Read the model definition and answer for the solid it produces. Units are mm, in the model's axes. A direction names the side the tool comes from. Coordinates: 2 decimals unless noted, no trailing zeros. Loops run counter-clockwise (first coordinate to the right, second up) from the corner with the lowest first, then second, coordinate; pieces in that order, holes last. Notation, with made-up numbers: (30, -39.75) - (88, -39.75) arc R33 cw to (88, -4.75) - close; hole circle Ø11 at (43, 10). An arc over 180 degrees is marked (long way). Use one line per item in the form item = value.
Autodesk Inventor part; units mm, degrees
ref_plane "Work Plane1" through (0, 0, 4.4125) normal (0, 0, 1) x (1, 0, 0)
ref_plane "YZ Plane" through (0, 0, 0) normal (1, 0, 0) x (0, 1, 0)
ref_plane "XZ Plane" through (0, 0, 0) normal (0, 1, 0) x (-1, 0, 0)
sketch "Sketch4" plane through (0, 0, 0) normal (0, 1, 0) x (-1, 0, 0)
  line L0 (0, 0) -> (6.5, 0) construction
  line L1 (6.5, 0) -> (6.5, -9.525)
  line L2 (6.5, -9.525) -> (0, -9.525)
  line L3 (0, -9.525) -> (0, 0)
  line L4 (0, -9.525) -> (19.05, -9.525)
  line L5 (19.05, -9.525) -> (19.05, 0) construction
  line L6 (19.05, 0) -> (0, 0)
  line L7 (0, 0) -> (0, -9.525) construction
  line L8 (19.05, 0) -> (16.9384, -9.525)
  line L9 (17.424, 0) -> (15.3123, -9.525)
  line L10 (15.6643, -7.9375) -> (6.5, -7.9375)
  line L11 (6.5, -7.9375) -> (7.5, -7.9375)
  line L12 (7.5, -7.9375) -> (7.5, -5.9375)
  line L13 (7.5, -5.9375) -> (6.5, -5.9375)
  line L14 (6.5, -5.9375) -> (6.5, -7.9375)
  line L15 (6.5, 0) -> (0, 0)
  line L16 (0, 0) -> (0, 6.35)
  line L17 (0, 6.35) -> (6.5, 6.35)
  line L18 (6.5, 6.35) -> (6.5, 0)
  line L19 (6.5, -3.175) -> (17.072, -3.175)
  line L20 (17.072, -3.175) -> (17.072, -1.5875) construction
  line L21 (17.072, -1.5875) -> (6.5, -1.5875)
  line L22 (6.5, -1.5875) -> (6.5, -3.175)
  line L23 (6.5, -3.175) -> (0, -3.175)
  line L24 (6.5, -1.5875) -> (7.5, -1.5875)
  line L25 (7.5, -1.5875) -> (7.5, 0.4125)
  line L26 (7.5, 0.4125) -> (6.5, 0.4125)
  line L27 (6.5, 0.4125) -> (6.5, -1.5875)
  line L28 (15.3123, -9.525) -> (15.3123, -3.175)
  point P0 (0, -3.175)
  point P1 (16.7201, -3.175)
  dimension "d28" = 6.5
  dimension "d30" = 19.05
  dimension "d31" = 9.525
  dimension "d32" = 12.5
  dimension "d33" = 1.5875
  dimension "d34" = 1.5875
  dimension "d36" = 1
  dimension "d37" = 2
  dimension "d53" = 6.35
  dimension "d54" = 1.5875
  dimension "d55" = 9.525
  dimension "d56" = 1
  dimension "d57" = 2
revolve "Revolution1" add sketch "Sketch4" angle 360 about axis through (0, 0, -9.525) along (0, 0, 1) contours L6 L25 L21 L1 | L1 L23 L3 L6 | L18 L26 L25 L6 | L6 L16 L17 L18 | L21 L9 L19 L1 | L6 L8 L4 L9 | L19 L9 L10 L28 | L10 L9 L28
sketch "Sketch5" plane through (0, 0, 0) normal (0, 0, 1) x (1, 0, 0)
  circle A0 centre (0, 0) radius 4.7625 construction
  line L0 (0, 0) -> (0, 4.7625) construction
  line L1 (2.7496, 4.7625) -> (5.4993, 0)
  line L2 (5.4993, 0) -> (2.7496, -4.7625)
  line L3 (2.7496, -4.7625) -> (-2.7496, -4.7625)
  line L4 (-2.7496, -4.7625) -> (-5.4993, 0)
  line L5 (-5.4993, 0) -> (-2.7496, 4.7625)
  line L6 (-2.7496, 4.7625) -> (2.7496, 4.7625)
  line L7 (-2.7496, 4.7625) -> (0, 0) construction
  arc A1 (-0.9165, 4.4712) -> (-2.6268, 4.5498) centre (-1.8331, 3.175) ccw
  arc A2 (-0.9165, 4.4712) -> (0, 4.1799) centre (0, 5.7674) ccw
  arc A3 (2.6268, 4.5498) -> (0.9165, 4.4712) centre (1.8331, 3.175) ccw
  arc A4 (0, 4.1799) -> (0.9165, 4.4712) centre (0, 5.7674) ccw
  arc A5 (-4.3304, 1.4418) -> (-5.2537, 0) centre (-3.6662, 0) ccw
  arc A6 (-4.3304, 1.4418) -> (-3.6199, 2.0899) centre (-4.9947, 2.8837) ccw
  arc A7 (-3.6199, 2.0899) -> (-3.4139, 3.0293) centre (-4.9947, 2.8837) ccw
  arc A8 (-2.6268, 4.5498) -> (-3.4139, 3.0293) centre (-1.8331, 3.175) ccw
  arc A9 (-3.4139, -3.0293) -> (-2.6268, -4.5498) centre (-1.8331, -3.175) ccw
  arc A10 (-3.4139, -3.0293) -> (-3.6199, -2.0899) centre (-4.9947, -2.8837) ccw
  arc A11 (-3.6199, -2.0899) -> (-4.3304, -1.4418) centre (-4.9947, -2.8837) ccw
  arc A12 (-5.2537, 0) -> (-4.3304, -1.4418) centre (-3.6662, 0) ccw
  arc A13 (0.9165, -4.4712) -> (2.6268, -4.5498) centre (1.8331, -3.175) ccw
  arc A14 (0.9165, -4.4712) -> (0, -4.1799) centre (0, -5.7674) ccw
  arc A15 (0, -4.1799) -> (-0.9165, -4.4712) centre (0, -5.7674) ccw
  arc A16 (-2.6268, -4.5498) -> (-0.9165, -4.4712) centre (-1.8331, -3.175) ccw
  arc A17 (4.3304, -1.4418) -> (5.2537, 0) centre (3.6662, 0) ccw
  arc A18 (4.3304, -1.4418) -> (3.6199, -2.0899) centre (4.9947, -2.8837) ccw
  arc A19 (3.6199, -2.0899) -> (3.4139, -3.0293) centre (4.9947, -2.8837) ccw
  arc A20 (2.6268, -4.5498) -> (3.4139, -3.0293) centre (1.8331, -3.175) ccw
  arc A21 (3.4139, 3.0293) -> (2.6268, 4.5498) centre (1.8331, 3.175) ccw
  arc A22 (3.4139, 3.0293) -> (3.6199, 2.0899) centre (4.9947, 2.8837) ccw
  arc A23 (3.6199, 2.0899) -> (4.3304, 1.4418) centre (4.9947, 2.8837) ccw
  arc A24 (5.2537, 0) -> (4.3304, 1.4418) centre (3.6662, 0) ccw
  point P0 (-1.8331, 4.7625)
  point P1 (-3.2079, 3.9688)
  point P2 (-5.041, 0.7937)
  point P3 (-5.041, -0.7938)
  point P4 (-3.2079, -3.9687)
  point P5 (-1.8331, -4.7625)
  point P6 (1.8331, -4.7625)
  point P7 (3.2079, -3.9687)
  point P8 (5.041, -0.7937)
  point P9 (5.041, 0.7937)
  point P10 (3.2079, 3.9687)
  point P11 (1.8331, 4.7625)
  dimension "d38" = 9.525
  dimension "d47" = 1.5875
  dimension "d48" = 1.5875
  dimension "d51" = 360
extrude "Extrusion4" cut sketch "Sketch5" along normal through all both and the other way through all
thicken "Thicken3" operation add thickness 0.0254 both sides no extend neighbours yes toward (0.9967573, -0.0804666, 0) faces at (-6.4789, 0.523, 2.3917)
ref_plane "Work Plane1" through (0, 0, 4.4125) normal (0, 0, 1) x (1, 0, 0)
sketch "Sketch6" plane through (0, 0, 4.4125) normal (0, 0, 1) x (1, 0, 0)
  circle A0 centre (0, 0) radius 6.2
  circle A1 centre (0, 0) radius 7.9375
  dimension "d43" = 12.4
  dimension "d44" = 15.875
extrude "Extrusion5" cut sketch "Sketch6" along normal blind 1.1
thicken "Thicken1" operation cut thickness 0.0127 both sides no extend neighbours yes toward (0.9505525, -0.2227193, 0.2164396) faces at (-17.8624, 4.1852, -3.175)
thicken "Thicken4" operation add thickness 0.0254 both sides no extend neighbours yes toward (0, 1, 0) faces at (0.9165, 4.7625, 3.175) (-4.5827, 1.5875, 3.175) (-4.5827, -1.5875, 0) (-0.9165, -4.7625, 0) (4.5827, -1.5875, 3.175) (4.5827, 1.5875, 0)
equation "\"d34\" = d33"
equation "\"d54\" = d34"
equation "\"d55\" = d31"
equation "\"d56\" = d36"
equation "\"d57\" = d37"
equation "\"d48\" = d47"
properties part number "Clutch" material "Stainless Steel"
Item 1: The part is cut by section B-B on z = 1.25. Give the vertices of the cut face in (x, y).
Results below:
outline = circle Ø12.95 at (0, 0); hole (-5.53, 0) - (-2.76, -4.79) - (2.76, -4.79) - (5.53, 0) - (2.76, 4.79) - (-2.76, 4.79) - close
Item 2: The part is cut by section C-C on z = -4.75. Give the vertices of the cut face in (x, y), plus the area to 3 significant figures.
Results below:
outline = circle Ø35.97 at (0, 0); hole circle Ø30.62 at (0, 0)
area = 279 mm²
Item 3: The part is cut by section D-D on z = -8.25. Give the vertices of the cut face in (x, y).
Results below:
outline = circle Ø34.42 at (0, 0); hole circle Ø30.62 at (0, 0)
Item 4: Find the intervals of material crossed by L1, parallel to X at y = 3, z = -0.75; L2, parallel to Z at x = 14, y = 6 (1 decimal); L3, parallel to Y at x = -3, z = 4.5, in increasing order.
Results below:
L1 = -18.63 to -16.99, -6.87 to -3.8, 3.8 to 6.87, 16.99 to 18.63
L2 = -3.2 to -1.6
L3 = -5.43 to -4.38, 4.38 to 5.43
Item 5: For a pull along Y with two mould halves and no side action, classify faces 1 (the flat face through (1, -5, 6.35)), 2 (the cylindrical face through (5.14, -3.94, 2.38)), 3 (the flat face through (-4.127, -2.427, 1.521)) as +Y half, -Y half, draft (parallel to the pull), parting line (faces both ways), or undercut.
Results below:
face_1 = draft
face_2 = parting line
face_3 = undercut
Item 6: Each of these flat-tipped pins is pushed along its axis until it touches: P1, Ø1, axis at x = -13, z = -3.5, coming from the +Y side; P2, Ø3, axis at x = -9.5, y = 11, coming from the +Z side; P3, Ø3, axis at x = -1, z = 0, coming from the -Y side. Where does it stop, or does it pass through?
Results below:
P1 = 13.34
P2 = -1.59
P3 = -19.04
Item 7: Which of the six approach directions +Z, -Z, +X, -X, +Y, -Y give full straight-line access (tool end or side, diameter ignored) to faces 4 (the flat face through (13, 9, -9.525)), 5 (the flat face through (6, 3, 0.412)), 6 (the flat face through (0, 4.788, 2)), 7 (the flat face through (4, -4, -3.175))?
Results below:
face_4 = -Z, +X, -X, +Y, -Y
face_5 = +Z
face_6 = +Z, -Z
face_7 = -Z
